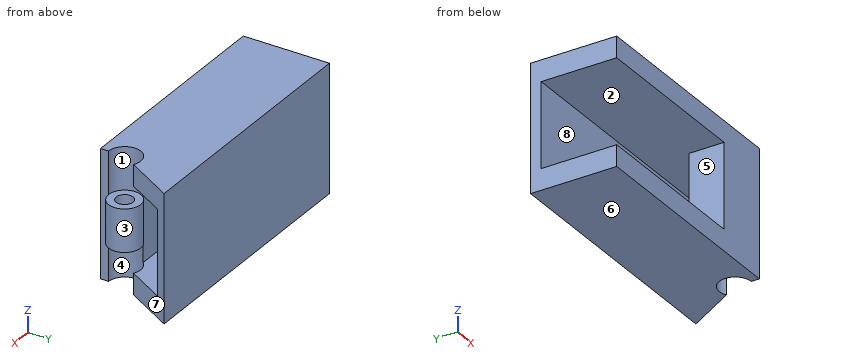
```python
from build123d import *

# Parameters (mm, degrees)
SKETCH_1_R          = 2
EXTRUDE_1_DEPTH     = 30
SKETCH_2_W          = 20
SKETCH_2_H          = 9.5
CUT_EXTRUDE_1_DEPTH = 70.293872581
EXTRUDE_START       = -30
SKETCH_3_R          = 3.79021957
SKETCH_3_R_2        = 2
EXTRUDE_2_DEPTH     = 30
CUT_EXTRUDE_START   = -10
SKETCH_4_R          = 3.79021957
SKETCH_4_R_2        = 2
CUT_EXTRUDE_2_DEPTH = 10
SKETCH_5_R          = 3.79021957
SKETCH_5_R_2        = 2
CUT_EXTRUDE_3_DEPTH = 10
SKETCH_6_W          = 20
SKETCH_6_H          = 8.329300022
CUT_EXTRUDE_4_DEPTH = 40


with BuildPart() as part:
    # 스케치1 → 보스-돌출1 (new body)
    # profile 1 of 6: a face of its own
    with BuildSketch(Plane.XY):
        with BuildLine():
            Line((-13.8475309, -1.196894222), (-7.287940278, 10.164650011))
            Line((-7.287940278, 10.164650011), (-37.287940278, 10.164650011))
            Line((-37.287940278, 10.164650011), (-37.287940278, -10.164650011))
            Line((-37.287940278, -10.164650011), (-15.742640685, -10.164650011))
            Line((-15.742640685, -10.164650011), (-15.742640685, -8.269540226))
            ThreePointArc((-15.742640685, -8.269540226), (-19.403711655, -3.498339646), (-13.8475309, -1.196894222))
        make_face()
    # profile 2 of 6: a face of its own
    with BuildSketch(Plane.XY):
        with BuildLine():
            ThreePointArc((-15.742640685, -8.269540226), (-12.081569715, -5.460301666), (-13.8475309, -1.196894222))
            ThreePointArc((-13.8475309, -1.196894222), (-19.403711655, -3.498339646), (-15.742640685, -8.269540226))
        make_face()
        with Locations((-15.742640685, -4.479320656)):
            Circle(SKETCH_1_R, mode=Mode.SUBTRACT)
    # profile 3 of 6: a face of its own
    with BuildSketch(Plane.XY):
        with Locations((-15.742640685, -4.479320656)):
            Circle(SKETCH_1_R)
    # profile 4 of 6: a face of its own
    with BuildSketch(Plane.XY):
        with BuildLine():
            Line((-7.287940278, -10.164650011), (-7.287940278, 10.164650011))
            Line((-7.287940278, 10.164650011), (-13.8475309, -1.196894222))
            ThreePointArc((-13.8475309, -1.196894222), (-12.081569715, -5.460301666), (-15.742640685, -8.269540226))
            Line((-15.742640685, -8.269540226), (-15.742640685, -10.164650011))
            Line((-15.742640685, -10.164650011), (-7.287940278, -10.164650011))
        make_face()
    # profile 5 of 6: a face of its own
    with BuildSketch(Plane.XY):
        with BuildLine():
            Line((7.433176247, 10.164650011), (-7.287940278, 10.164650011))
            Line((-7.287940278, 10.164650011), (-7.287940278, -10.164650011))
            Line((-7.287940278, -10.164650011), (15.887876654, -10.164650011))
            Line((15.887876654, -10.164650011), (15.887876654, -8.269540226))
            ThreePointArc((15.887876654, -8.269540226), (19.548947624, -5.460301666), (17.782986439, -1.196894222))
            ThreePointArc((17.782986439, -1.196894222), (15.887876654, -0.689101086), (13.992766869, -1.196894222))
            Line((13.992766869, -1.196894222), (7.433176247, 10.164650011))
        make_face()
        with Locations((15.887876654, -4.479320656)):
            Circle(SKETCH_1_R, mode=Mode.SUBTRACT)
    # profile 6 of 6: a face of its own
    with BuildSketch(Plane.XY):
        with BuildLine():
            Line((24.342577061, 10.164650011), (7.433176247, 10.164650011))
            Line((7.433176247, 10.164650011), (13.992766869, -1.196894222))
            ThreePointArc((13.992766869, -1.196894222), (15.887876654, -0.689101086), (17.782986439, -1.196894222))
            Line((17.782986439, -1.196894222), (24.342577061, 10.164650011))
        make_face()
    extrude(amount=EXTRUDE_1_DEPTH)

    # 스케치2 → 컷-돌출1 (cut, through all)
    with BuildSketch(Plane.ZY.offset(37.287940278)):
        with Locations((15, 2.914650011)):
            Rectangle(SKETCH_2_W, SKETCH_2_H)
    extrude(amount=-CUT_EXTRUDE_1_DEPTH, mode=Mode.SUBTRACT)

    # 스케치3 → 보스-돌출2 (add)
    with BuildSketch(Plane.XY.offset(30).offset(EXTRUDE_START)):
        with Locations((15.887876654, -4.479320656)):
            Circle(SKETCH_3_R)
        with Locations((15.887876654, -4.479320656)):
            Circle(SKETCH_3_R_2, mode=Mode.SUBTRACT)
    extrude(amount=EXTRUDE_2_DEPTH)

    # 스케치4 → 컷-돌출2 (cut)
    with BuildSketch(Plane.XY.offset(30).offset(CUT_EXTRUDE_START)):
        with Locations((15.887876654, -4.479320656)):
            Circle(SKETCH_4_R)
        with Locations((15.887876654, -4.479320656)):
            Circle(SKETCH_4_R_2, mode=Mode.SUBTRACT)
    extrude(amount=CUT_EXTRUDE_2_DEPTH, mode=Mode.SUBTRACT)

    # 스케치5 → 컷-돌출3 (cut)
    with BuildSketch(Plane(origin=(0, 0, 0), x_dir=(-1, 0, 0), z_dir=(0, 0, -1))):
        with Locations((-15.887876654, -4.479320656)):
            Circle(SKETCH_5_R)
        with Locations((-15.887876654, -4.479320656)):
            Circle(SKETCH_5_R_2, mode=Mode.SUBTRACT)
    extrude(amount=-CUT_EXTRUDE_3_DEPTH, mode=Mode.SUBTRACT)

    # 스케치6 → 컷-돌출4 (cut)
    with BuildSketch(Plane.ZY.offset(37.287940278)):
        with Locations((15, -6)):
            Rectangle(SKETCH_6_W, SKETCH_6_H)
    extrude(amount=-CUT_EXTRUDE_4_DEPTH, mode=Mode.SUBTRACT)


solid = part.part
```
Model file for the job. Use its own axes, mm. Face numbers are marked on the shaded views. A direction names the side the tool comes from. Coordinates: 2 decimals unless noted, no trailing zeros. Write each loop counter-clockwise with the first axis right and the second up, starting at its lowest first coordinate (ties: lowest second). Pieces come first, ordered by that corner, then holes. Notation, with made-up numbers: (11, 40.5) - (59, 40.5) arc R26 cw to (59, 64.5) - close; hole circle Ø2 at (75.5, -33.5). An arc over 180 degrees is marked (long way). Use a Markdown table: item, result. Add a question column.
Item 1: Band-saw the part on A-A, the plane x = -5. Write the cut outline in (y, z), and give its area (3 significant figures).
Item 2: 3-axis set-ups, long thin cutter, end or side, ignore diameter. For the marked faces 1, 2, 3, 4 and 5: which of +Z, -Z, +X, -X, +Y, -Y reach the whole face in a straight line?
Item 3: Two-plate mould, pull along Z, no slides. Class the marked faces 6, 7 and 8: pulls with the +Z half, pulls with the -Z half, needs draft (parallel to the pull), parting line crosses it, or undercut.
Item 4: Drill centre lines: line 1 along Z through (x, y) = (-33, -0.75); line 2 along Y through (x, z) = (10.5, 11.25); line 3 along Y through (x, z) = (-12.5, 11). Where is each one in solid material? Low to high.
Item 5: Drop flat-ended pins along their axis: pin 1 (1.5 mm diameter, centred on x = 14, y = -6, fed in from +Z); pin 2 (3 mm diameter, centred on x = -26.5, z = 18, fed in from -Y); pin 3 (6 mm diameter, centred on y = -4.5, z = 20.5, fed in from +X). Give the stop position or say it passes through.
Item 6: Band-saw the part on D-D, the plane z = 18.5. Write the cut outline in (x, y), and give its area (3 significant figures).
Item 7: Band-saw the part on C-C, the plane z = 8.5. Write the cut outline in (x, y), and give its area (3 significant figures).
Item 8: Band-saw the part on B-B, the plane y = -3.25. Write the cut outline in (x, z).
A:
| question | item | result |
|---|---|---|
| 1 | outline | (-10.16, 0) - (10.16, 0) - (10.16, 30) - (-10.16, 30) - (-10.16, 25) - (7.66, 25) - (7.66, 5) - (-10.16, 5) - close |
| 1 | area | 253 mm² |
| 2 | face 1 | +Z |
| 2 | face 2 | -X |
| 2 | face 3 | none |
| 2 | face 4 | -Z |
| 2 | face 5 | -X, -Y |
| 3 | face 6 | pulls with the -Z half |
| 3 | face 7 | needs draft |
| 3 | face 8 | undercut |
| 4 | line 1 | z = 0 to 5, 25 to 30 |
| 4 | line 2 | y = -10.16 to -1.84, 7.66 to 10.16 |
| 4 | line 3 | y = 7.66 to 10.16 |
| 5 | pin 1 | stops at z = 20 |
| 5 | pin 2 | stops at y = 7.66 |
| 5 | pin 3 | stops at x = 19.68 |
| 6 | outline | (-37.29, 7.66) - (22.9, 7.66) - (24.34, 10.16) - (-37.29, 10.16) - close; (2.71, -10.16) - (15.89, -10.16) - (15.89, -8.27) arc R3.79 ccw (long way) to (13.17, -1.84) - (2.71, -1.84) - close; hole circle Ø4 at (15.89, -4.48) |
| 6 | area | 274 mm² |
| 7 | outline | (-37.29, 7.66) - (22.9, 7.66) - (24.34, 10.16) - (-37.29, 10.16) - close; (2.71, -10.16) - (15.89, -10.16) - (15.89, -8.27) arc R3.79 cw to (13.17, -1.84) - (2.71, -1.84) - close |
| 7 | area | 242 mm² |
| 8 | outline | (-37.29, 0) - (12.3, 0) - (12.3, 10) - (14.31, 10) - (14.31, 20) - (12.3, 20) - (12.3, 30) - (-37.29, 30) - (-37.29, 25) - (2.71, 25) - (2.71, 5) - (-37.29, 5) - close; (17.47, 10) - (19.47, 10) - (19.47, 20) - (17.47, 20) - close |
